Geometry: final body of the model. Coordinates: model frame, mm. Round coordinates to 2 decimals unless told otherwise and drop trailing zeros. Loops run counter-clockwise (first coordinate to the right, second up) from the corner with the lowest first, then second, coordinate; pieces in that order, holes last. Notation, with made-up numbers: (2.25, 67.5) - (34.25, 67.5) arc R25 cw to (34.25, 103.5) - close; hole circle Ø7 at (78, 36.5). An arc over 180 degrees is marked (long way). Use CSV: the item, a comma, the result in double quotes.
Autodesk Inventor part; units mm, degrees
ref_plane "YZ Plane" through (0, 0, 0) normal (1, 0, 0) x (0, 1, 0)
ref_plane "XZ Plane" through (0, 0, 0) normal (0, 1, 0) x (-1, 0, 0)
ref_plane "XY Plane" through (0, 0, 0) normal (0, 0, 1) x (1, 0, 0)
sketch "Sketch1" plane through (0, 0, 0) normal (0, 1, 0) x (-1, 0, 0)
  arc A0 (13.9253, -19.1836) -> (13.9253, 18.9664) centre (13.9253, -0.1086) ccw
  arc A1 (-13.9253, 18.9664) -> (-13.9253, -19.1836) centre (-13.9253, -0.1086) ccw
  line L0 (33, 0) -> (-33, 0) construction
  line L1 (13.9253, 18.9664) -> (-13.9253, 18.9664)
  line L2 (14.2135, -19.1836) -> (-13.9253, -19.1836)
  line L3 (-13.9253, -0.1086) -> (-13.9253, 18.9664) construction
  line L4 (-13.9253, -0.1086) -> (-13.9253, -19.1836) construction
  line L5 (13.9253, 18.9664) -> (13.9253, -19.1836) construction
  circle A2 centre (13.9253, -0.1086) radius 3.05
  circle A3 centre (-13.9253, -0.1086) radius 3.05
  point P0 (0, 0)
  point P1 (0, 0)
  dimension "d0" = 38.15
  dimension "d1" = 66
  dimension "d4" = 27.8506
  dimension "d7" = 6.1
extrude "Extrusion1" add sketch "Sketch1" along normal blind 3.8
properties part number "hinge" material "Steel, Carbon"
Item 1: Section D-D on x = 15. Return the cut outline in (y, z).
Final values:
outline,"(0, -19.15) - (3.8, -19.15) - (3.8, -2.96) - (0, -2.96) - close; (0, 2.75) - (3.8, 2.75) - (3.8, 18.94) - (0, 18.94) - close"
Item 2: Pin query (flat end, axial travel): P1, Ø2, axis at y = 3, z = 4.5, coming from the +X side. Return the tip coordinate at first contact, or that it passes through.
Final values:
P1,"stops at x = 32.66"
Item 3: Mould query, pull axis X, two halves, no side actions, for faces 1 (the cylindrical face through (32.996, 1.873, -0.528)), 2 (the cylindrical face through (16.972, 1.873, -0.243)), 3 (the flat face through (0, 0, 0)). Classes: released by +X, released by -X, zero draft, split by the parting line, or undercut.
Final values:
face 1,"released by +X"
face 2,"undercut"
face 3,"zero draft"
Item 4: Section A-A on z = 2. Return the cut outline in (x, y), plus the area to 3 significant figures.
Final values:
outline,"(-32.88, 0) - (-16.13, 0) - (-16.13, 3.8) - (-32.88, 3.8) - close; (-11.72, 0) - (11.72, 0) - (11.72, 3.8) - (-11.72, 3.8) - close; (16.13, 0) - (32.88, 0) - (32.88, 3.8) - (16.13, 3.8) - close"
area,"216 mm²"
Item 5: Material intervals for line 1 (X direction, y = 3.55, z = -2.5); line 2 (X direction, y = 2.5, z = 2.5); line 3 (X direction, y = 1.5, z = 17.5), sorted ascending.
Final values:
line 1,"x = -32.85 to -15.82, -12.03 to 12.03, 15.82 to 32.85"
line 2,"x = -32.82 to -15.51, -12.34 to 12.34, 15.51 to 32.82"
line 3,"x = -21.26 to 21.26"
Item 6: Section C-C on y = 2.75. Return the cut outline in (x, z) (3 decimals), plus the area to 3 significant figures.
Final values:
outline,"(-13.925, -19.184) - (13.925, -19.184) arc R19.075 ccw to (13.925, 18.966) - (-13.925, 18.966) arc R19.075 ccw to start; hole circle Ø6.1 at (-13.925, -0.109); hole circle Ø6.1 at (13.925, -0.109)"
area,"2,150 mm²"
Item 7: Section B-B on x = -12. Return the cut outline in (y, z), plus the area to 3 significant figures.
Final values:
outline,"(0, -19.18) - (3.8, -19.18) - (3.8, -2.47) - (0, -2.47) - close; (0, 2.26) - (3.8, 2.26) - (3.8, 18.97) - (0, 18.97) - close"
area,"127 mm²"
